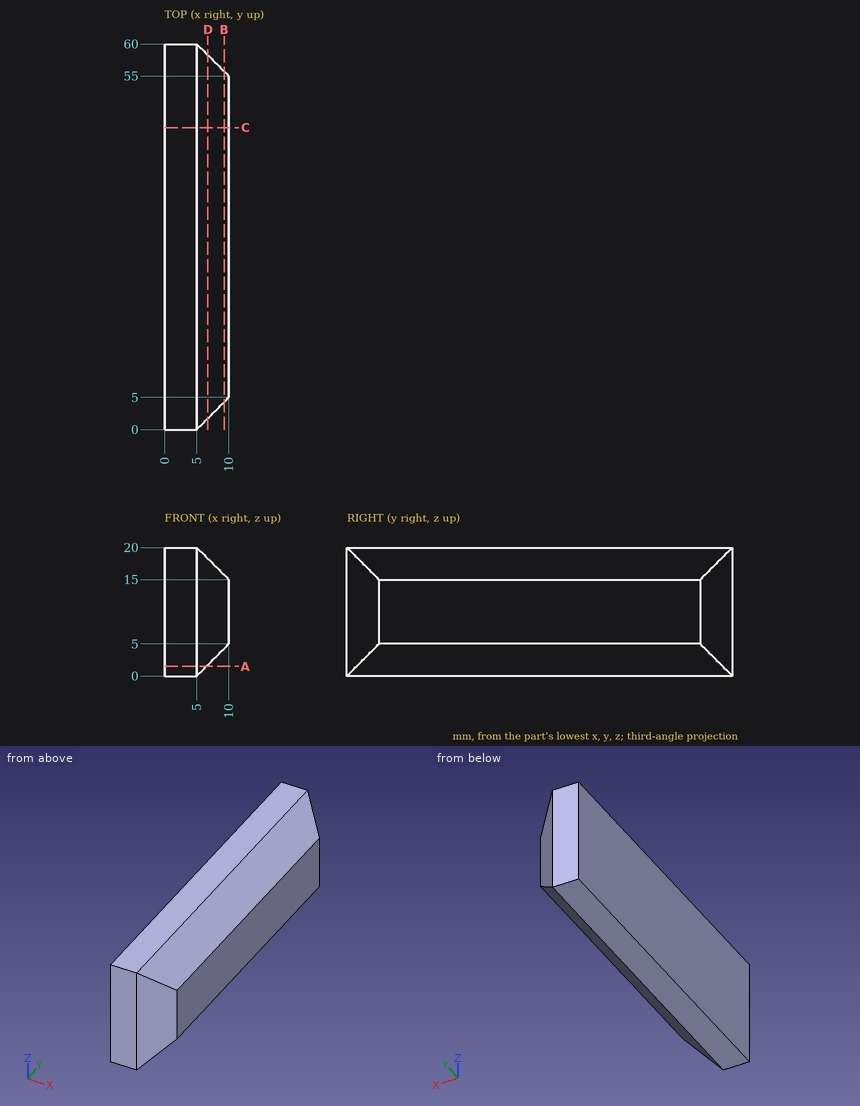
For this review, use the dimensioned drawing (mm, ordinates from the lowest corner) and the shaded views. Give positions to 0.01 mm unless a question says otherwise; leave off trailing zeros. Write each loop counter-clockwise with the first axis right and the second up, starting at its lowest first coordinate (ties: lowest second). Pieces come first, ordered by that corner, then holes.
(1) Consider section B-B, the plane x = 9.25. Give the boundary of the cut face in (y, z), and give its area (3 significant figures).
(2) Consider section D-D, the plane x = 6.75. Give the boundary of the cut face in (y, z).
(3) For P1, Ø3, axis at x = 8, y = 14.5, coming from the +Z side; P2, Ø1.5, axis at y = 18.5, z = 16, coming from the +X side, all flat-tipped, find the tip position at first contact; note any pin that passes through.
(4) Consider section A-A, the plane z = 1.5. Give the boundary of the cut face in (x, y).
(5) To check wall thickness, follow L1, parallel to X at y = 22, z = 4; L2, parallel to Z at x = 9.25, y = 38.5; L3, parallel to Y at x = 5.25, z = 15.5. State the ranges of each line that lie inside material, in increasing order.
(6) Consider section C-C, the plane y = 47. Give the boundary of the cut face in (x, z).
Returned:
1. outline: (4.25, 4.25) - (55.75, 4.25) - (55.75, 15.75) - (4.25, 15.75) - close
1. area: 592 mm2
2. outline: (1.75, 1.75) - (58.25, 1.75) - (58.25, 18.25) - (1.75, 18.25) - close
3. P1: stops at z = 18.5
3. P2: stops at x = 9.75
4. outline: (0, 0) - (5, 0) - (6.5, 1.5) - (6.5, 58.5) - (5, 60) - (0, 60) - close
5. L1: x = 0 to 9
5. L2: z = 4.25 to 15.75
5. L3: y = 0.25 to 59.75
6. outline: (0, 0) - (5, 0) - (10, 5) - (10, 15) - (5, 20) - (0, 20) - close
